Source: three-view drawing plus pictorial views. Frame: mm from the lowest corner of the part. A direction names the side the tool comes from. Give positions to 0.01 mm unless a question says otherwise; leave off trailing zeros. Write each loop counter-clockwise with the first axis right and the second up, starting at its lowest first coordinate (ties: lowest second). Pieces come first, ordered by that corner, then holes. Notation, with made-up numbers: (-28, -30) -> (0, -30) arc R7 ccw to (0, -20) -> close; hole circle Ø10 at (-38.75, 42.25). An arc over 180 degrees is marked (long way). Answer in a Markdown table with one row per item. Add a question column.
Item 1: First-contact query: P1, Ø1.5, axis at x = 52.5, y = 43, coming from the +Z side; P2, Ø12, axis at x = 22, z = 59, coming from the -Y side; P3, Ø2, axis at y = 42.5, z = 39, coming from the -X side; P4, Ø5, axis at y = 41.5, z = 25, coming from the -X side. Flat tips, straight axial feed; report the tip coordinate or a pass-through.
Item 2: Section query B-B on z = 40. Output: boundary loops of the cut face in (x, y), plus the area to 3 significant figures.
Item 3: Section query C-C on y = 36. Output: boundary loops of the cut face in (x, z), plus the area to 3 significant figures.
Item 4: Access query for the marked faces 1 and 2. Directions: +Z, -Z, +X, -X, +Y, -Y. A direction counts if a zero-diameter tool reaches every point of the face in a straight line with its end or side. Return the directions, or none.
Item 5: Section query D-D on y = 44. Output: boundary loops of the cut face in (x, z), plus the area to 3 significant figures.
Item 6: Section query A-A on x = 52. Output: boundary loops of the cut face in (y, z), plus the area to 3 significant figures.
Item 7: Material intervals for probe 1 along Y at (x, z) = (20.5, 50); probe 2 along Y at (x, z) = (66.5, 74); probe 3 along Z at (x, y) = (47.5, 46), sorted ascending. Write a range as from..to.
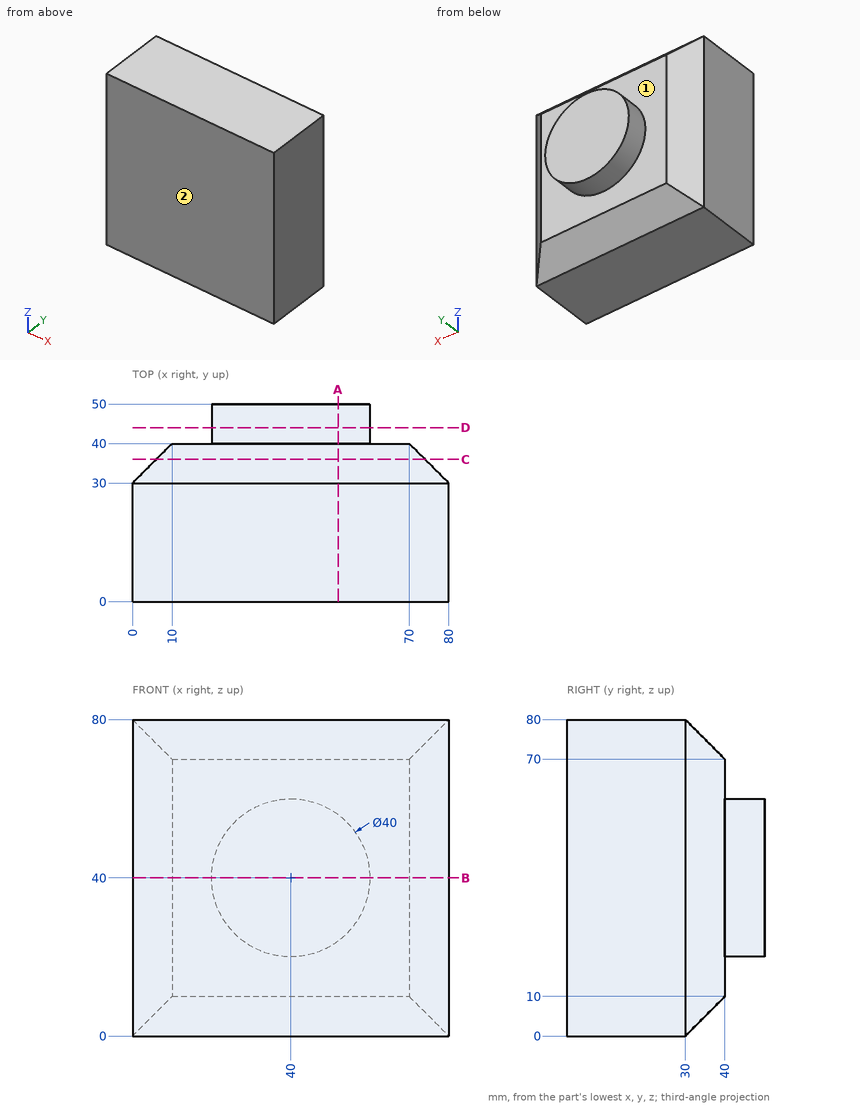
Findings below:
| question | item | result |
|---|---|---|
| 1 | P1 | stops at z = 56.18 |
| 1 | P2 | stops at y = 0 |
| 1 | P3 | stops at x = 20 |
| 1 | P4 | stops at x = 9 |
| 2 | outline | (0, 0) -> (80, 0) -> (80, 30) -> (70, 40) -> (60, 40) -> (60, 50) -> (20, 50) -> (20, 40) -> (10, 40) -> (0, 30) -> close |
| 2 | area | 3,500 mm^2 |
| 3 | outline | (6, 6) -> (74, 6) -> (74, 74) -> (6, 74) -> close |
| 3 | area | 4,620 mm^2 |
| 4 | face 1 | +Y |
| 4 | face 2 | +Z, -Z, +X, -X, -Y |
| 5 | outline | circle Ø40 at (40, 40) |
| 5 | area | 1,260 mm^2 |
| 6 | outline | (0, 0) -> (30, 0) -> (40, 10) -> (40, 24) -> (50, 24) -> (50, 56) -> (40, 56) -> (40, 70) -> (30, 80) -> (0, 80) -> close |
| 6 | area | 3,420 mm^2 |
| 7 | probe 1 | y = 0..40 |
| 7 | probe 2 | y = 0..36 |
| 7 | probe 3 | z = 21.46..58.54 |
